Can you work these out from the drawing? Everything is in mm from the part's minimum corner. Round coordinates to 2 decimals unless told otherwise and drop trailing zeros. Order: outer loops, then holes, each group sorted by start corner. A loop starts at its lowest first (then second) coordinate and runs counter-clockwise, first axis right, second up. Notation, with made-up numbers: (-17.5, -17) - (41.5, -17) arc R21 cw to (41.5, -1) - close; hole circle Ø9 at (-18.5, -21). An arc over 180 degrees is marked (long way). Answer as a JSON object with one key per item and string values.
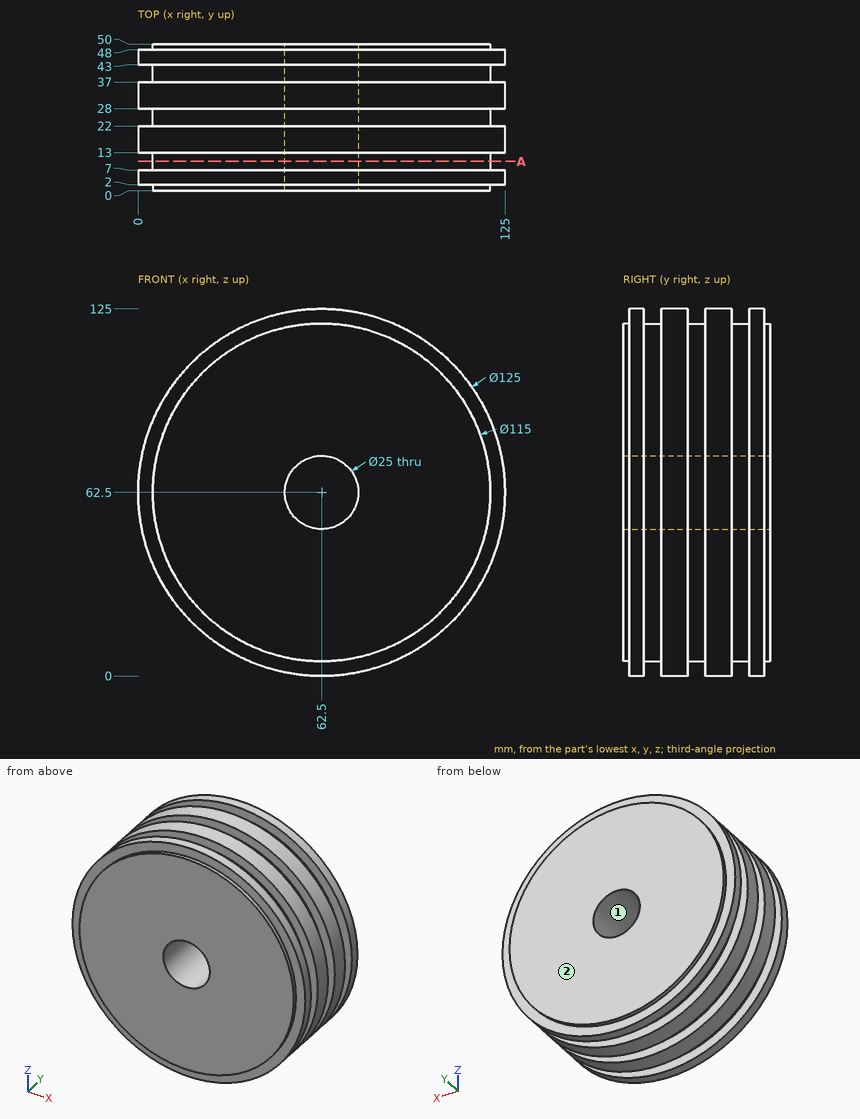
1. If I drill on L1, parallel to Y at x = 32, z = 115; L2, parallel to X at y = 20, z = 62.5; L3, parallel to X at y = 38, z = 62.5, over which ranges is the centre line in solid material (lowest first)? Write a range as [from, to].
Responses:
{"L1": "[2, 7], [13, 22], [28, 37], [43, 48]", "L2": "[0, 50], [75, 125]", "L3": "[5, 50], [75, 120]"}
2. For P1, Ø8, axis at x = 103, y = 31, coming from the +Z side; P2, Ø10, axis at x = 90.5, y = 18, coming from the -Z side; P3, Ø1, axis at y = 29.5, z = 56, coming from the +X side, each with a flat end and sliding along its axis, tell me the tip position at first contact or that it passes through.
Responses:
{"P1": "z = 113.23", "P2": "z = 4.39", "P3": "x = 124.71"}
3. Thinking about a two-plate mould opening in Z: for the marked faces 1 and 2, which applies, pulls with the +Z half, pulls with the -Z half, needs draft (parallel to the pull), parting line crosses it, or undercut?
Responses:
{"face 1": "undercut", "face 2": "needs draft"}
4. Imagine slicing it at A-A (y = 10). List the corners of the cut face in (x, z) for me, plus the area to 3 significant figures.
Responses:
{"outline": "circle Ø115 at (62.5, 62.5); hole circle Ø25 at (62.5, 62.5)", "area": "9,900 mm2"}
